Read the model definition and answer for the solid it produces. Units are mm, in the model's axes. A direction names the side the tool comes from. Give positions to 0.01 mm unless a question says otherwise; leave off trailing zeros. Loops run counter-clockwise (first coordinate to the right, second up) from the corner with the lowest first, then second, coordinate; pieces in that order, holes last. Notation, with made-up numbers: (0.25, 6.25) - (23.25, 6.25) arc R25 ccw to (23.25, 34.25) - close; hole circle Ø11 at (56, 46). An arc over 180 degrees is marked (long way). Use a Markdown table: item, result. Add a question column.
Item 1: A cutting plane is placed at B-B (z = -10). Determine the outline of the cut face in (x, y).
Item 2: A cutting plane is placed at D-D (x = 11.5). Determine the outline of the cut face in (y, z).
Item 3: A cutting plane is placed at A-A (z = 8). Determine the outline of the cut face in (x, y), plus the area to 4 significant figures.
Item 4: Which of the six approach directions +Z, -Z, +X, -X, +Y, -Y give full straight-line access (tool end or side, diameter ignored) to faces 4 (the face through (44, 22, 5.5)), 5 (the face through (44, 23, -12.5)), 6 (the face through (-44, 18, 15.5)), 7 (the face through (1, 3, 0)), 8 (the face through (45.25, 11, 0))?
Item 5: A cutting plane is placed at C-C (y = 18.75). Determine the outline of the cut face in (x, z).
Item 6: Each of these flat-tipped pins is pushed along its axis until it touches: P1, Ø5, axis at x = 17, z = 13, coming from the +Y side; P2, Ø3.5, axis at x = 43.5, z = -15.5, coming from the +Y side. Where does it stop, or does it pass through?
Item 7: For a pull along Z with two mould halves and no side action, classify faces 1 (the face through (44, 17, 14)), 2 (the face through (1, 15, -31.5)), 3 (the face through (-1, 15, 31.5)) as +Z half, -Z half, draft (parallel to the pull), parting line (faces both ways), or undercut.
Item 8: Consider probe 1 along X at (y, z) = (28.8, 29.5); probe 2 along Z at (x, y) = (43.25, 26.8); probe 3 along Z at (x, y) = (-7.5, 21.75). Determine where each line is inside the solid, lowest interval first. Write a range as [from, to].
Autodesk Inventor part; units mm, degrees
ref_plane "YZ Plane" through (0, 0, 0) normal (1, 0, 0) x (0, 1, 0)
ref_plane "XZ Plane" through (0, 0, 0) normal (0, 1, 0) x (-1, 0, 0)
ref_plane "XY Plane" through (0, 0, 0) normal (0, 0, 1) x (1, 0, 0)
sketch "Sketch1" plane through (0, 0, 0) normal (0, 1, 0) x (-1, 0, 0)
  line L0 (45.25, 31.5) -> (-45.25, 31.5)
  line L1 (-45.25, 31.5) -> (-45.25, -31.5)
  line L2 (-45.25, -31.5) -> (45.25, -31.5)
  line L3 (45.25, -31.5) -> (45.25, 31.5)
  line L4 (45.25, 31.5) -> (-45.25, -31.5) construction
  line L5 (-45.25, 31.5) -> (45.25, -31.5) construction
  point P0 (0, 0)
  dimension "d0" = 63
  dimension "d1" = 90.5
extrude "Extrusion1" add sketch "Sketch1" along normal blind 3
sketch "Sketch2" plane through (0, 3, 0) normal (0, 1, 0) x (1, 0, 0)
  line L0 (-42.25, -28.5) -> (42.25, -28.5)
  line L1 (42.25, -28.5) -> (42.25, 28.5)
  line L2 (42.25, 28.5) -> (-42.25, 28.5)
  line L3 (-42.25, 28.5) -> (-42.25, -28.5)
  line L4 (-42.25, -28.5) -> (42.25, 28.5) construction
  line L5 (42.25, -28.5) -> (-42.25, 28.5) construction
  line L6 (45.25, -31.5) -> (45.25, 31.5)
  line L7 (-45.25, -31.5) -> (45.25, -31.5)
  line L8 (45.25, -31.5) -> (45.25, 31.5)
  line L9 (45.25, 31.5) -> (-45.25, 31.5)
  line L10 (-45.25, 31.5) -> (-45.25, -31.5)
  line L11 (-45.25, -31.5) -> (45.25, 31.5) construction
  line L12 (45.25, -31.5) -> (-45.25, 31.5) construction
  point P0 (0, 0)
  point P1 (45.25, -31.5)
  dimension "d4" = 57
  dimension "d5" = 84.5
extrude "Extrusion2" add sketch "Sketch2" along normal blind 27
sketch "Sketch3" plane through (0, 30, 0) normal (0, 1, 0) x (1, 0, 0)
  circle A0 centre (-43.25, 29.5) radius 0.75
  line L0 (45.25, 31.5) -> (-45.25, 31.5)
  line L1 (-45.25, 31.5) -> (-45.25, -31.5)
  circle A1 centre (-43.25, -29.5) radius 0.75
  line L2 (-45.25, -31.5) -> (45.25, -31.5)
  circle A2 centre (43.25, -29.5) radius 0.75
  line L3 (45.25, -31.5) -> (45.25, 31.5)
  circle A3 centre (43.25, 29.5) radius 0.75
  point P0 (0, 0)
  dimension "d8" = 2
  dimension "d9" = 2
  dimension "d10" = 1.5
  dimension "d11" = 2
  dimension "d12" = 2
  dimension "d13" = 1.5
  dimension "d14" = 2
  dimension "d15" = 2
  dimension "d16" = 1.5
  dimension "d17" = 2
  dimension "d18" = 2
  dimension "d19" = 1.5
extrude "Extrusion3" cut sketch "Sketch3" against normal blind 5 contours A0 | A1 | A2 | A3
sketch "Sketch5" plane through (-45.25, 0, -31.5) normal (-1, 0, 0) x (0, 0, 1)
  line L0 (16, 14) -> (47, 14)
  line L1 (47, 14) -> (47, 22)
  line L2 (47, 22) -> (16, 22)
  line L3 (16, 22) -> (16, 14)
  line L4 (0, 0) -> (63, 0)
  line L5 (0, 0) -> (0, 30)
  point P0 (31.5, 0)
  dimension "d23" = 14
  dimension "d24" = 8
  dimension "d25" = 31
  dimension "d26" = 16
extrude "Extrusion4" cut sketch "Sketch5" against normal blind 3
sketch "Sketch6" plane through (45.25, 0, 31.5) normal (1, 0, 0) x (0, 0, -1)
  line L0 (44, 30) -> (56, 30)
  line L1 (56, 30) -> (56, 17)
  line L2 (56, 17) -> (44, 17)
  line L3 (44, 17) -> (44, 30)
  line L4 (0, 0) -> (63, 0)
  line L5 (63, 0) -> (63, 30)
  line L6 (9, 26) -> (26, 26)
  line L7 (26, 26) -> (26, 17)
  line L8 (26, 17) -> (9, 17)
  line L9 (9, 17) -> (9, 26)
  line L10 (0, 0) -> (0, 30)
  point P0 (31.5, 0)
  dimension "d30" = 17
  dimension "d31" = 13
  dimension "d32" = 12
  dimension "d33" = 7
  dimension "d34" = 9
  dimension "d35" = 17
  dimension "d36" = 17
  dimension "d37" = 9
extrude "Extrusion5" cut sketch "Sketch6" against normal blind 3
properties part number "remoteswitchbox"
Geometry says:
| question | item | result |
|---|---|---|
| 1 | outline | (-45.25, 0) - (45.25, 0) - (45.25, 30) - (42.25, 30) - (42.25, 3) - (-42.25, 3) - (-42.25, 14) - (-45.25, 14) - close; (-45.25, 22) - (-42.25, 22) - (-42.25, 30) - (-45.25, 30) - close |
| 2 | outline | (0, -31.5) - (30, -31.5) - (30, -28.5) - (3, -28.5) - (3, 28.5) - (30, 28.5) - (30, 31.5) - (0, 31.5) - close |
| 3 | outline | (-45.25, 0) - (45.25, 0) - (45.25, 17) - (42.25, 17) - (42.25, 3) - (-42.25, 3) - (-42.25, 14) - (-45.25, 14) - close; (-45.25, 22) - (-42.25, 22) - (-42.25, 30) - (-45.25, 30) - close; (42.25, 26) - (45.25, 26) - (45.25, 30) - (42.25, 30) - close |
| 3 | area | 382.5 mm² |
| 4 | face 4 | +X |
| 4 | face 5 | +X, +Y |
| 4 | face 6 | -X |
| 4 | face 7 | +Y |
| 4 | face 8 | +Z, -Z, +X, +Y, -Y |
| 5 | outline | (-45.25, -31.5) - (45.25, -31.5) - (45.25, -24.5) - (42.25, -24.5) - (42.25, -28.5) - (-42.25, -28.5) - (-42.25, -15.5) - (-45.25, -15.5) - close; (-45.25, 15.5) - (-42.25, 15.5) - (-42.25, 28.5) - (42.25, 28.5) - (42.25, 22.5) - (45.25, 22.5) - (45.25, 31.5) - (-45.25, 31.5) - close; (42.25, -12.5) - (45.25, -12.5) - (45.25, 5.5) - (42.25, 5.5) - close |
| 6 | P1 | y = 3 |
| 6 | P2 | y = 17 |
| 7 | face 1 | undercut |
| 7 | face 2 | -Z half |
| 7 | face 3 | +Z half |
| 8 | probe 1 | [-45.25, -44], [-42.5, 42.5], [44, 45.25] |
| 8 | probe 2 | [-31.5, -30.25], [-28.75, -24.5], [-12.5, 28.75], [30.25, 31.5] |
| 8 | probe 3 | [-31.5, -28.5], [28.5, 31.5] |
